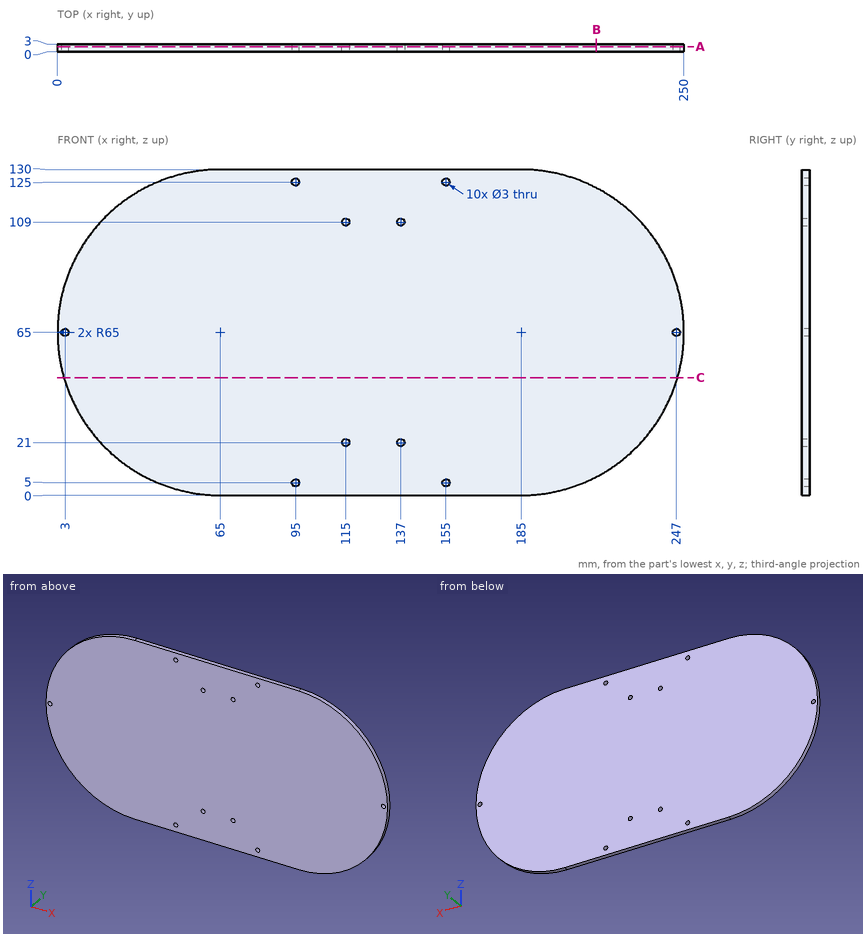
Answer from the drawing. Dimensions are ordinates in mm from the lowest x, y and z of the part. Coordinates: 2 decimals unless noted, no trailing zeros. Loops run counter-clockwise (first coordinate to the right, second up) from the corner with the lowest first, then second, coordinate; pieces in that order, holes last.
Q1. Consider probe 1 along Z at (x, y) = (95, 1.3); probe 2 along Z at (x, y) = (115, 1.6); probe 3 along X at (y, z) = (1.1, 109). Determine where each line is inside the solid, lowest interval first.
Q2. The part is cut by section B-B on x = 215. Write down the section's boundary in (y, z), and give its area (3 significant figures).
Q3. Each of these flat-tipped pins is pushed along its axis until it touches: pin 1 Ø2.5 at (x, z) = (137, 21) entering from -Y; pin 2 Ø1.5 at (x, y) = (33, 2) entering from +Z. Where does it stop, or does it pass through?
Q4. The part is cut by section A-A on y = 1.95. Give the number of separate pieces and of enclosed holes in the cut face, and give its area (3 significant figures).
Q5. The part is cut by section C-C on z = 47. Write down the section's boundary in (x, y).
Results below:
1. probe 1: z = 0 to 3.5, 6.5 to 123.5, 126.5 to 130
1. probe 2: z = 0 to 19.5, 22.5 to 107.5, 110.5 to 130
1. probe 3: x = 17.16 to 113.5, 116.5 to 135.5, 138.5 to 232.84
2. outline: (0, 7.34) - (3, 7.34) - (3, 122.66) - (0, 122.66) - close
2. area: 346 mm2
3. pin 1: passes through
3. pin 2: stops at z = 122
4. separate pieces: 1
4. enclosed holes: 10
4. area: 28,800 mm2
5. outline: (2.54, 0) - (247.46, 0) - (247.46, 3) - (2.54, 3) - close
